Geometry check sheet. Reference: drawing and pictorial views, mm from the part's lowest x, y, z. A direction names the side the tool comes from. Give positions to 0.01 mm unless a question says otherwise; leave off trailing zeros. Write each loop counter-clockwise with the first axis right and the second up, starting at its lowest first coordinate (ties: lowest second). Pieces come first, ordered by that corner, then holes. Notation, with made-up numbers: (-13.75, 36.25) -> (27.25, 36.25) arc R12 ccw to (27.25, 49.25) -> close; hole circle Ø6 at (-5.75, 12.25). An arc over 180 degrees is marked (long way). Use a Markdown table: item, result. Add a question column.
1. Cross-section at D-D (y = 14.5). Enter the section's corners in (x, z).
2. Cross-section at A-A (y = 10). Enter the section's corners in (x, z).
3. Release check for a two-part mould opening along X. For the marked faces 1 and 2 record: released by +X, released by -X, zero draft, split by the parting line, or undercut.
4. Set-up check for the marked faces 3 and 4: record each of +Z, -Z, +X, -X, +Y, -Y from which the full face is reachable in a straight line by a thin tool's end or side.
5. Scan lines: probe 1 along Y at (x, z) = (6.45, 9.55); probe 2 along X at (y, z) = (5.75, 8); probe 3 along X at (y, z) = (8.25, 6.25) (1 decimal). Record each from-to range of solid material in increasing order. Write a range as [from, to].
6. Cross-section at C-C (x = 7). Enter the section's corners in (y, z).
7. Gauge pin test, flat ends, axial feed: P1, Ø4, axis at x = 2, y = 11, coming from the +Z side; P2, Ø6, axis at x = 11, y = 12, coming from the +Z side. Record the tip position at first contact, or that the pin passes through.
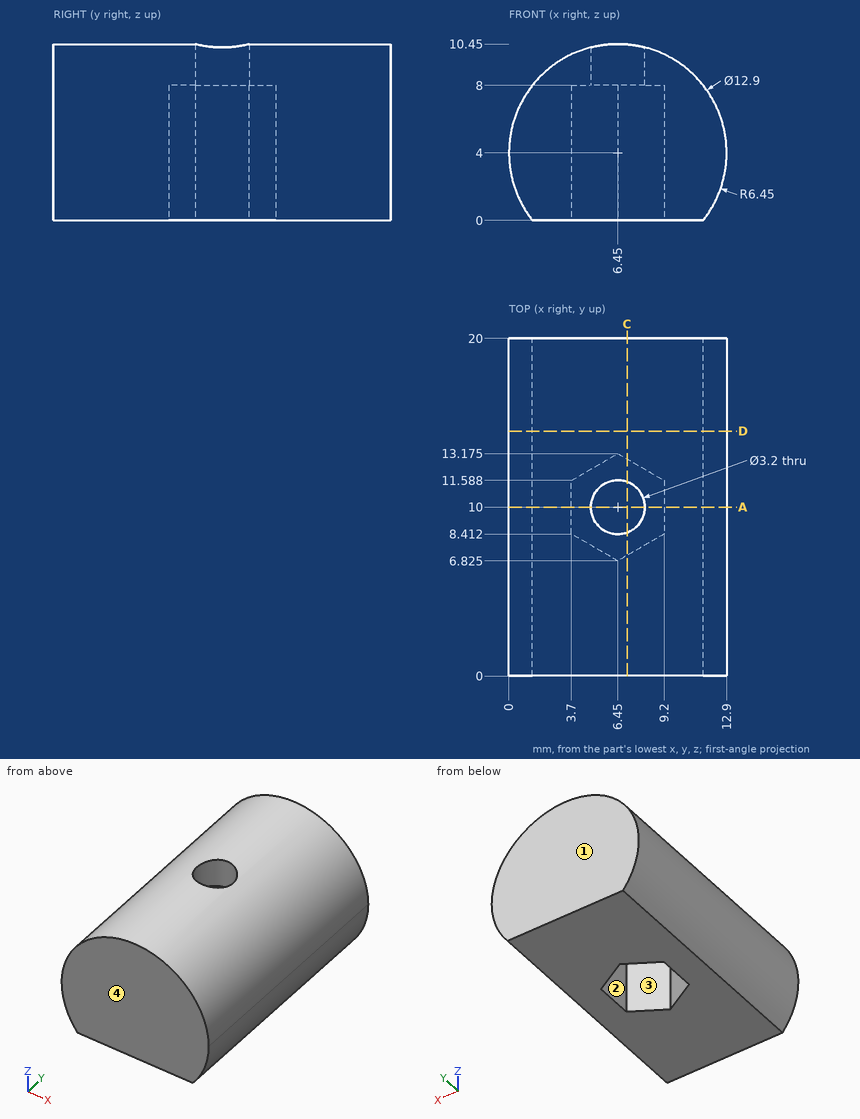
Worked answers:
| question | item | result |
|---|---|---|
| 1 | outline | (1.39, 0) -> (11.51, 0) arc R6.45 ccw (long way) to start |
| 2 | outline | (1.39, 0) -> (3.7, 0) -> (3.7, 8) -> (4.85, 8) -> (4.85, 10.25) arc R6.45 ccw to start; (8.05, 8) -> (9.2, 8) -> (9.2, 0) -> (11.51, 0) arc R6.45 ccw to (8.05, 10.25) -> close |
| 3 | face 1 | zero draft |
| 3 | face 2 | undercut |
| 4 | face 3 | -Z |
| 4 | face 4 | +Z, -Z, +X, -X, -Y |
| 5 | probe 1 | y = [0, 8.4], [11.6, 20] |
| 5 | probe 2 | x = [1.39, 11.51] |
| 5 | probe 3 | x = [0.4, 4], [8.9, 12.5] |
| 6 | outline | (0, 0) -> (7.14, 0) -> (7.14, 8) -> (8.5, 8) -> (8.5, 10.43) -> (0, 10.43) -> close; (11.5, 8) -> (12.86, 8) -> (12.86, 0) -> (20, 0) -> (20, 10.43) -> (11.5, 10.43) -> close |
| 7 | P1 | stops at z = 9.97 |
| 7 | P2 | stops at z = 10.26 |
